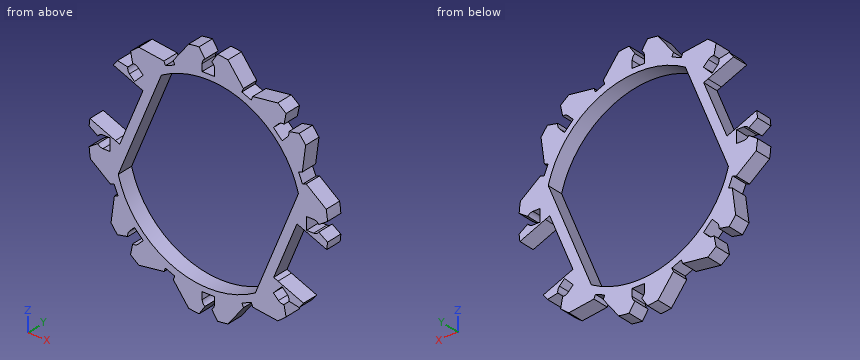
from build123d import *

# Parameters (mm, degrees)
SKETCH1_R           = 54.55
BOSS_EXTRUDE1_DEPTH = 7.5
SKETCH2_R           = 42.5
CUT_EXTRUDE1_DEPTH  = 78.509063986
CUT_EXTRUDE2_DEPTH  = 78.509063986
CUT_EXTRUDE6_DEPTH  = 78.509063986
CIRPATTERN1_COUNT   = 8
CIRPATTERN2_COUNT   = 8
CUT_EXTRUDE7_DEPTH  = 78.279736538
BOSS_EXTRUDE2_DEPTH = 7.5


with BuildPart() as part:
    # Sketch1 → Boss-Extrude1 (new body)
    with BuildSketch(Plane(origin=(0, 0, 0), x_dir=(1, 0, 0), z_dir=(0, 1, 0))):
        with Locations(Location((0, 0, 0), (0, 0, 270))):
            Circle(SKETCH1_R)
    extrude(amount=BOSS_EXTRUDE1_DEPTH)

    # Sketch2 → Cut-Extrude1 (cut, through all)
    with BuildSketch(Plane(origin=(0, 7.5, 0), x_dir=(1, 0, 0), z_dir=(0, 1, 0))):
        with Locations(Location((0, 0, 0), (0, 0, 270))):
            Circle(SKETCH2_R)
    extrude(amount=-CUT_EXTRUDE1_DEPTH, mode=Mode.SUBTRACT)

    # Sketch3 → Cut-Extrude2 (cut, through all)
    with BuildSketch(Plane(origin=(0, 7.5, 0), x_dir=(1, 0, 0), z_dir=(0, 1, 0))):
        with BuildLine():
            Line((-2.8, -48.082), (-2.8, -44.832))
            Line((-2.8, -44.832), (2.8, -44.832))
            Line((2.8, -44.832), (2.8, -48.082))
            ThreePointArc((2.8, -48.082), (2.46937954, -49.401910863), (1.555596652, -50.410114914))
            Line((1.555596652, -50.410114914), (4.212915889, -54.387074197))
            ThreePointArc((4.212915889, -54.387074197), (0, -54.55), (-4.212915889, -54.387074197))
            Line((-4.212915889, -54.387074197), (-1.555596652, -50.410114914))
            ThreePointArc((-1.555596652, -50.410114914), (-2.46937954, -49.401910863), (-2.8, -48.082))
        make_face()
    cut_extrude2 = extrude(amount=-CUT_EXTRUDE2_DEPTH, mode=Mode.SUBTRACT)

    # Sketch9 → Cut-Extrude6 (cut, through all)
    with BuildSketch(Plane(origin=(0, 7.5, 0), x_dir=(1, 0, 0), z_dir=(0, 1, 0))):
        with BuildLine():
            Line((-20.257229317, -42.895088115), (-31.690865911, -44.400354929))
            ThreePointArc((-31.690865911, -44.400354929), (-20.875381236, -50.397628498), (-8.98696587, -53.804618245))
            Line((-8.98696587, -53.804618245), (-16.007383468, -44.655431904))
            Line((-16.007383468, -44.655431904), (-15.318553289, -42.992448745))
            Line((-15.318553289, -42.992448745), (-19.568399139, -41.232104956))
            Line((-19.568399139, -41.232104956), (-20.257229317, -42.895088115))
        make_face()
    cut_extrude6 = extrude(amount=-CUT_EXTRUDE6_DEPTH, mode=Mode.SUBTRACT)

    # CirPattern1: Cut-Extrude2 ×8 about axis
    cirpattern1_axis = Axis((0, 0, 0), (0, 1, 0))
    for i in range(1, CIRPATTERN1_COUNT):
        add(cut_extrude2.rotate(cirpattern1_axis, i * 360 / CIRPATTERN1_COUNT), mode=Mode.SUBTRACT)

    # CirPattern2: Cut-Extrude6 ×8 about axis, 2 skipped
    cirpattern2_axis = Axis((0, 10.872185225, 0), (0, -1, 0))
    add([cut_extrude6.rotate(cirpattern2_axis, i * 360 / CIRPATTERN2_COUNT) for i in range(1, CIRPATTERN2_COUNT) if i not in (1, 5)], mode=Mode.SUBTRACT)

    # Sketch10 → Cut-Extrude7 (cut, through all)
    with BuildSketch(Plane.XZ):
        Polygon((-42.422842704, 2.559768914), (-31.807509711, 28.187449796), (-46.056303911, 34.089493601), (-56.671636904, 8.461812719), align=None)
    cut_extrude7 = extrude(amount=-CUT_EXTRUDE7_DEPTH, mode=Mode.SUBTRACT)

    # Sketch11 → Boss-Extrude2 (add, through all)
    with BuildSketch(Plane.XZ):
        with BuildLine():
            Line((-42.422842704, 2.559768914), (-40.442805118, 1.739610492))
            Line((-40.442805118, 1.739610492), (-29.827472125, 27.367291374))
            Line((-29.827472125, 27.367291374), (-31.807509711, 28.187449796))
            ThreePointArc((-31.807509711, 28.187449796), (-26.965878836, 32.849526307), (-21.449800959, 36.689999166))
            Line((-21.449800959, 36.689999166), (-41.111046925, -10.776447499))
            ThreePointArc((-41.111046925, -10.776447499), (-42.295878596, -4.160367025), (-42.422842704, 2.559768914))
        make_face()
    boss_extrude2 = extrude(amount=-BOSS_EXTRUDE2_DEPTH)

    # Mirror1: Cut-Extrude7, Boss-Extrude2 across plane
    add(cut_extrude7.mirror(Plane(origin=(0, 0, 0), x_dir=(0.38268343236508123, 0, 0.9238795325112903), z_dir=(0.9238795325112903, 0, -0.38268343236508123))), mode=Mode.SUBTRACT)
    add(boss_extrude2.mirror(Plane(origin=(0, 0, 0), x_dir=(0.38268343236508123, 0, 0.9238795325112903), z_dir=(0.9238795325112903, 0, -0.38268343236508123))))


solid = part.part
Check sheet for the modelled part. Datum: model origin and axes. Units: mm. Give positions to 0.01 mm unless a question says otherwise; leave off trailing zeros. Loops run counter-clockwise (first coordinate to the right, second up) from the corner with the lowest first, then second, coordinate; pieces in that order, holes last. Notation, with made-up numbers: M 45,-34.75 L 95,-34.75 A6 ccw 95,-29.75 Z; hole C 76,60 d7. An arc over 180 degrees is marked long. Use a Markdown table: item, result. Add a question column.
Q1. Scan lines: line 1 along Z through (x, y) = (1, 5.5); line 2 along X through (y, z) = (6.25, -7); line 3 along X through (y, z) = (6, 15.5). Record each from-to range of solid material in increasing order. Write a range as [from, to].
Q2. Go/stop test with flat-tipped pins: pin 1 (2.5 mm diameter, centred on y = 2, z = -45.5, fed in from -X); pin 2 (1.6 mm diameter, centred on x = 46.5, y = 5, fed in from -Z); pin 3 (3 mm diameter, centred on y = 4.5, z = 1.5, fed in from -X). Record where each tip stops, or that it passes through.
Q3. Sectioned sample at A-A, the plane x = 7. Record the cut outline in (y, z), then the cut area to 3 significant figures.
Q4. Sectioned sample at B-B, the plane z = 22. Record the cut outline in (x, y).
Verdict:
| question | item | result |
|---|---|---|
| 1 | line 1 | [-44.83, -42.49], [42.49, 44.83] |
| 1 | line 2 | [-54.1, -39.55], [33.75, 38.26], [53.14, 54.1] |
| 1 | line 3 | [-34.74, -30.23], [39.57, 42.92], [43.43, 45.32] |
| 2 | pin 1 | x = -31.9 |
| 2 | pin 2 | z = -4.58 |
| 2 | pin 3 | x = -52.57 |
| 3 | outline | M 0,-54.1 L 7.5,-54.1 L 7.5,-41.92 L 0,-41.92 Z; M 0,41.92 L 7.5,41.92 L 7.5,54.1 L 0,54.1 Z |
| 3 | area | 183 mm^2 |
| 4 | outline | M -32.05,0 L -27.53,0 L -27.53,7.5 L -32.05,7.5 Z; M 36.36,0 L 43.12,0 L 43.12,7.5 L 36.36,7.5 Z |
